Model file for the job. Use its own axes, mm. A direction names the side the tool comes from. Coordinates: 2 decimals unless noted, no trailing zeros. Order: outer loops, then holes, each group sorted by start corner. A loop starts at its lowest first (then second) coordinate and runs counter-clockwise, first axis right, second up. Notation, with made-up numbers: M -8.75,76.25 L 30.25,76.25 A14 ccw 30.25,82.25 Z; hole C 6,26.5 d1. An arc over 180 degrees is marked long. Return JSON: item names as keys, results as strings.
Autodesk Inventor part; units mm, degrees
ref_plane "YZ Plane" through (0, 0, 0) normal (1, 0, 0) x (0, 1, 0)
ref_plane "XZ Plane" through (0, 0, 0) normal (0, 1, 0) x (-1, 0, 0)
ref_plane "XY Plane" through (0, 0, 0) normal (0, 0, 1) x (1, 0, 0)
sketch "Sketch1" plane through (0, 0, 0) normal (0, 0, 1) x (1, 0, 0)
  line L0 (0, 0) -> (-88.9, 0)
  line L1 (-88.9, 0) -> (-88.9, 38.1)
  line L2 (-88.9, 38.1) -> (0, 38.1)
  line L3 (0, 38.1) -> (0, 0)
  circle A0 centre (-69.85, 19.05) radius 10.5029
  dimension "d0" = 88.9
  dimension "d1" = 38.1
  dimension "d2" = 21.0058
  dimension "d3" = 19.05
  dimension "d4" = 19.05
extrude "Extrusion1" add sketch "Sketch1" along normal blind 3.175
sketch "Sketch2" plane through (0, 0, 3.175) normal (0, 0, 1) x (1, 0, 0)
  line L0 (-88.9, 38.1) -> (-88.9, 0)
  line L1 (0, 0) -> (0, 38.1)
  line L2 (-88.9, 38.1) -> (0, 38.1)
  line L3 (0, 38.1) -> (0, 0)
  line L4 (0, 0) -> (-88.9, 0)
  line L5 (-88.9, 0) -> (-88.9, 38.1)
  line L6 (-3.175, 34.925) -> (-85.725, 34.925)
  line L7 (-85.725, 34.925) -> (-85.725, 3.175)
  line L8 (-85.725, 3.175) -> (-3.175, 3.175)
  line L9 (-3.175, 3.175) -> (-3.175, 34.925)
  dimension "d7" = 3.175
extrude "Extrusion2" add sketch "Sketch2" along normal blind 28.575
sketch "Sketch3" plane through (0, 0, 3.175) normal (0, 0, 1) x (1, 0, 0)
  line L0 (-3.175, 34.925) -> (-3.175, 3.175)
  line L1 (-85.725, 3.175) -> (-3.175, 3.175)
  line L2 (-3.175, 34.925) -> (-49.8348, 34.925)
  line L3 (-49.8348, 34.925) -> (-49.8348, 3.175)
  line L4 (-49.8348, 3.175) -> (-3.175, 3.175)
  line L5 (-3.175, 3.175) -> (-3.175, 34.925)
  point P0 (0, 0)
  dimension "d10" = 46.6598
extrude "Extrusion3" add sketch "Sketch3" along normal blind 12.7
sketch "Sketch4" plane through (0, 0, 0) normal (1, 0, 0) x (0, 0, -1)
  circle A0 centre (-22.225, 19.05) radius 3.81
  line L0 (-31.75, 0) -> (-31.75, 38.1)
  point P0 (0, 0)
  dimension "d13" = 7.62
  dimension "d14" = 9.525
extrude "Extrusion4" cut sketch "Sketch4" against normal blind 19.05
properties part number "escbox"
Item 1: Wall check: line 1 (Z direction, x = -1, y = 19); line 2 (X direction, y = 13, z = 9) (3 decimals); line 3 (Y direction, x = -33, z = 26.5) (3 decimals). Give the ranges that are in metal, low to high.
Check result:
{"line 1": "z = 0 to 18.42, 26.03 to 31.75", "line 2": "x = -88.9 to -85.725, -49.835 to 0", "line 3": "y = 0 to 3.175, 34.925 to 38.1"}
Item 2: Drop flat-ended pins along their axis: pin 1 Ø9.5 at (x, y) = (-35.5, 26.5) entering from +Z (3 decimals); pin 2 Ø16 at (x, y) = (-67, 25) entering from +Z (3 decimals). Give the stop position or say it passes through.
Check result:
{"pin 1": "stops at z = 15.875", "pin 2": "stops at z = 3.175"}
Item 3: Pull direction Y, two halves, no side cores. Call faces 4 (the flat face through (-48, 2, 31.75)), 5 (the flat face through (-49.835, 19, 9)), 6 (the flat face through (-44, 0, 16)): +Y half, -Y half, draft (parallel to the pull), parting line (faces both ways), or undercut.
Check result:
{"face 4": "draft", "face 5": "undercut", "face 6": "-Y half"}
Item 4: Saw through at D-D (y = 6.5). Write the cut outline in (x, z) (3 decimals).
Check result:
{"outline": "M -88.9,0 L 0,0 L 0,31.75 L -3.175,31.75 L -3.175,15.875 L -49.835,15.875 L -49.835,3.175 L -85.725,3.175 L -85.725,31.75 L -88.9,31.75 Z"}
Item 5: Saw through at C-C (y = 12). Write the cut outline in (x, z) (3 decimals), and give its area (3 significant figures).
Check result:
{"outline": "M -88.9,0 L -77.635,0 L -77.635,3.175 L -85.725,3.175 L -85.725,31.75 L -88.9,31.75 Z; M -62.065,0 L 0,0 L 0,31.75 L -3.175,31.75 L -3.175,15.875 L -49.835,15.875 L -49.835,3.175 L -62.065,3.175 Z", "area": "1,010 mm2"}
Item 6: 3-axis set-ups, long thin cutter, end or side, ignore diameter. For faces 1 (the flat face through (0, 19, 16)), 2 (the flat face through (-3.175, 19, 27)), 3 (the cylindrical face through (-1.565, 22.828, 22.721)): which of +Z, -Z, +X, -X, +Y, -Y reach the whole face in a straight line?
Check result:
{"face 1": "+Z, -Z, +X, +Y, -Y", "face 2": "+Z", "face 3": "+X"}
Item 7: Saw through at A-A (y = 19.05). Write the cut outline in (x, z) (3 decimals), and give its area (3 significant figures).
Check result:
{"outline": "M -88.9,0 L -80.353,0 L -80.353,3.175 L -85.725,3.175 L -85.725,31.75 L -88.9,31.75 Z; M -59.347,0 L 0,0 L 0,18.415 L -3.175,18.415 L -3.175,15.875 L -49.835,15.875 L -49.835,3.175 L -59.347,3.175 Z; M -3.175,26.035 L 0,26.035 L 0,31.75 L -3.175,31.75 Z", "area": "965 mm2"}
Item 8: Saw through at B-B (x = -69.85). Write the cut outline in (y, z) (3 decimals), and give its area (3 significant figures).
Check result:
{"outline": "M 0,0 L 8.547,0 L 8.547,3.175 L 3.175,3.175 L 3.175,31.75 L 0,31.75 Z; M 29.553,0 L 38.1,0 L 38.1,31.75 L 34.925,31.75 L 34.925,3.175 L 29.553,3.175 Z", "area": "236 mm2"}
